The listing builds one solid part. Answer for the finished solid, in the listing's coordinates (mm). Face numbers are marked on the shaded views. A direction names the side the tool comes from. Round coordinates to 2 decimals unless told otherwise and drop trailing zeros. Order: outer loops, then holes, each group sorted by start corner. A loop starts at its lowest first (then second) coordinate and runs counter-clockwise, first axis right, second up. Notation, with made-up numbers: (30, -8) - (86, -8) arc R23 ccw to (86, 31) - close; hole circle Ø1 at (-32, 55.5). An arc over 180 degrees is marked (long way). Write item = value, one per line.
from build123d import *

# Parameters (mm, degrees)
SKICA1_R                 = 34.5
P_IDAT_VYSUNUT_M1_DEPTH  = 48
SKICA2_R                 = 4
ODEBRAT_VYSUNUT_M1_DEPTH = 40
SKICA3_R                 = 5
ODEBRAT_VYSUNUT_M2_DEPTH = 69.443407279
KRUHOV_POLE1_COUNT       = 3


with BuildPart() as part:
    # Skica1 → Přidat vysunutím1 (new body)
    with BuildSketch(Plane.XY):
        Circle(SKICA1_R)
    extrude(amount=P_IDAT_VYSUNUT_M1_DEPTH)

    # Skica2 → Odebrat vysunutím1 (cut)
    with BuildSketch(Plane.XY.offset(48)):
        with Locations((0, 20.207259422)):
            Circle(SKICA2_R)
        with Locations((17.5, -10.103629711)):
            Circle(SKICA2_R)
        with Locations((-17.5, -10.103629711)):
            Circle(SKICA2_R)
    extrude(amount=-ODEBRAT_VYSUNUT_M1_DEPTH, mode=Mode.SUBTRACT)

    # Skica3 → Odebrat vysunutím2 (cut, through all)
    with BuildSketch(Plane(origin=(0, 0, 0), x_dir=(1, 0, 0), z_dir=(0, 1, 0))):
        with Locations(Location((0, -29, 0), (0, 0, 270))):
            Circle(SKICA3_R)
    odebrat_vysunut_m2 = extrude(amount=-ODEBRAT_VYSUNUT_M2_DEPTH, mode=Mode.SUBTRACT)

    # Kruhové pole1: Odebrat vysunutím2 ×3 about axis
    kruhov_pole1_axis = Axis((0, 0, 48), (0, 0, -1))
    for i in range(1, KRUHOV_POLE1_COUNT):
        add(odebrat_vysunut_m2.rotate(kruhov_pole1_axis, i * 360 / KRUHOV_POLE1_COUNT), mode=Mode.SUBTRACT)


solid = part.part
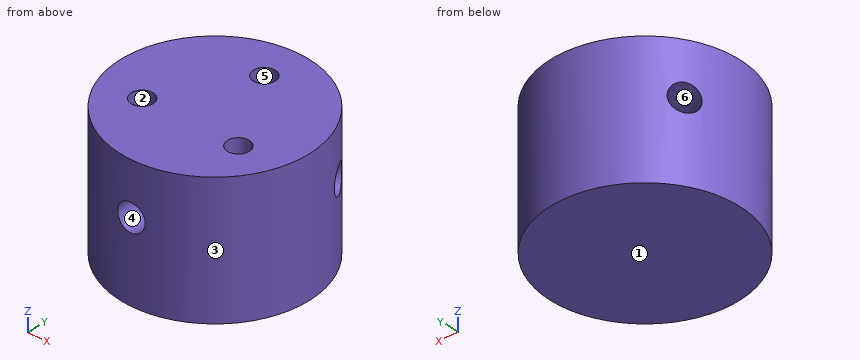
Q1. Flat-ended cylindrical pins translate along their axes: P1, Ø9, axis at x = 0, z = 29, coming from the +Y side; P2, Ø4, axis at x = -16, z = 20, coming from the -Y side; P3, Ø3, axis at y = -16.5, z = 10, coming from the -X side; P4, Ø4, axis at y = 2, z = 27, coming from the +X side. Find the tip coordinate at first contact, or state that the pin passes through.
Model answer:
P1 = 34.5
P2 = -31.53
P3 = -31.07
P4 = 34.5
Q2. Section D-D on y = -18 is taken. Determine the outline of the cut face in (x, z).
Model answer:
outline = (-29.43, 0) - (29.43, 0) - (29.43, 48) - (-29.43, 48) - close; hole circle Ø10 at (0, 29)
Q3. Find the intervals of material crossed by line 1 (Z direction, x = 0, y = -19); line 2 (Y direction, x = -17.5, z = 26.5); line 3 (Y direction, x = 0, z = 36.5), in increasing order. Write a range as from..to.
Model answer:
line_1 = 0..24, 34..48
line_2 = -29.73..-14.1, -6.1..5.1, 15.1..29.73
line_3 = -34.5..16.21, 24.21..34.5
Q4. For the marked faces 4, 5 and 6, determine the directions among +Z, -Z, +X, -X, +Y, -Y from which every point of the face is accessible in a straight line to the end or side of a thin tool.
Model answer:
face_4 = -Y
face_5 = +Z
face_6 = none
Q5. Section C-C on z = 4.5 is taken. Determine the outline of the cut face in (x, y).
Model answer:
outline = circle Ø69 at (0, 0)
Q6. Section B-B on y = -11 is taken. Determine the outline of the cut face in (x, z), then the cut area to 3 significant figures.
Model answer:
outline = (-32.7, 0) - (32.7, 0) - (32.7, 48) - (21.4, 48) - (21.4, 8) - (13.6, 8) - (13.6, 48) - (-13.6, 48) - (-13.6, 8) - (-21.4, 8) - (-21.4, 48) - (-32.7, 48) - close; hole circle Ø10 at (0, 29)
area = 2,440 mm^2
Q7. Section A-A on z = 29 is taken. Determine the outline of the cut face in (x, y).
Model answer:
outline = (-32.06, 12.74) arc R34.5 ccw to (-5, -34.14) - (-5, -2.89) - close; (-27.06, 21.4) - (0, 5.77) - (27.06, 21.4) arc R34.5 ccw to start; (5, -34.14) arc R34.5 ccw to (32.06, 12.74) - (5, -2.89) - close; hole circle Ø8 at (-17.5, -10.1); hole circle Ø8 at (0, 20.21); hole circle Ø8 at (17.5, -10.1)
Q8. Determine the mould class of the marked faces 1, 2 and 3 for opening direction Y: released by +Y, released by -Y, zero draft, split by the parting line, or undercut.
Model answer:
face_1 = zero draft
face_2 = undercut
face_3 = split by the parting line
